Can you work these out from the drawing? Everything is in mm from the part's minimum corner. Give positions to 0.01 mm unless a question says otherwise; leave off trailing zeros. Write each loop counter-clockwise with the first axis right and the second up, starting at its lowest first coordinate (ties: lowest second). Pieces come first, ordered by that corner, then holes. Notation, with made-up numbers: (4.25, -15.75) -> (17.25, -15.75) arc R24 cw to (17.25, -4.75) -> close; hole circle Ø5 at (-4.75, -2). An arc over 180 degrees is marked (long way). Return JSON: item names as keys, results as strings.
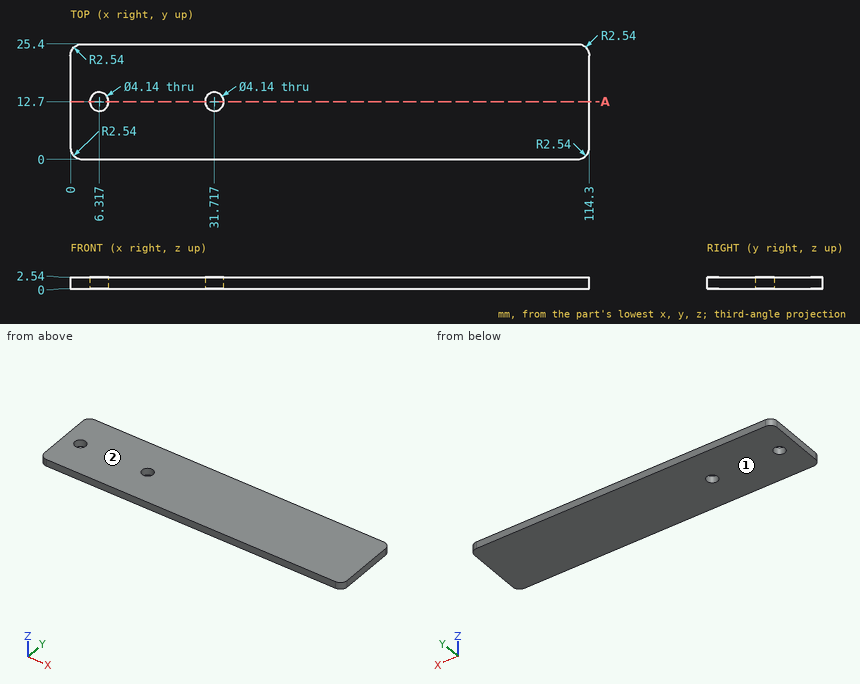
1. If I drill on line 1 (X direction, y = 12.7, z = 0.8); line 2 (X direction, y = 1.5, z = 1.75), over which ranges is the centre line in solid material (lowest first)? Write a range as [from, to].
Taken from the geometry:
{"line 1": "x = [0, 4.25], [8.39, 29.65], [33.79, 114.3]", "line 2": "x = [0.22, 114.08]"}
2. If we mould it in two halves opening along Z, with no side actions, what happens to the marked faces 1 and 2? For each: released by +Z, released by -Z, zero draft, split by the parting line, or undercut.
Taken from the geometry:
{"face 1": "released by -Z", "face 2": "released by +Z"}
3. Suppose I cut it at A-A, the plane y = 12.7. List the corners of the cut face in (x, z) for me.
Taken from the geometry:
{"outline": "(0, 0) -> (4.25, 0) -> (4.25, 2.54) -> (0, 2.54) -> close; (8.39, 0) -> (29.65, 0) -> (29.65, 2.54) -> (8.39, 2.54) -> close; (33.79, 0) -> (114.3, 0) -> (114.3, 2.54) -> (33.79, 2.54) -> close"}
4. For pin 1 Ø5 at (x, y) = (31.72, 12.7) entering from +Z; pin 2 Ø3.5 at (x, y) = (6.32, 12.7) entering from -Z, each with a flat end and sliding along its axis, tell me the tip position at first contact or that it passes through.
Taken from the geometry:
{"pin 1": "stops at z = 2.54", "pin 2": "passes through"}
